```python
from build123d import *

# Parameters (mm, degrees)
SKETCH1_R           = 25.4
BOSS_EXTRUDE1_DEPTH = 10.9
SKETCH4_OUTSIDE_W   = 67.332
SKETCH4_OUTSIDE_H   = 67.332
SKETCH4_OUTSIDE_R   = 23.9
CUT_EXTRUDE3_DEPTH  = 3
SHELL2_T            = -1.5
SKETCH2_R           = 1.7
CUT_EXTRUDE1_DEPTH  = 38.538380359
FILLET1_R           = 3
SKETCH3_R           = 22.5
CUT_EXTRUDE2_DEPTH  = 1.1


with BuildPart() as part:
    # Sketch1 → Boss-Extrude1 (new body)
    with BuildSketch(Plane(origin=(0, 0, 0), x_dir=(1, 0, 0), z_dir=(0, 1, 0))):
        with Locations(Location((0, 0, 0), (0, 0, 270))):
            Circle(SKETCH1_R)
    extrude(amount=BOSS_EXTRUDE1_DEPTH)

    # Sketch4 outside → Cut-Extrude3 (cut)
    with BuildSketch(Plane.XZ):
        Rectangle(SKETCH4_OUTSIDE_W, SKETCH4_OUTSIDE_H)
        with Locations(Location((0, 0, 0), (0, 0, 270))):
            Circle(SKETCH4_OUTSIDE_R, mode=Mode.SUBTRACT)
    extrude(amount=-CUT_EXTRUDE3_DEPTH, mode=Mode.SUBTRACT)

    # Shell2
    shell2_openings = [part.faces().sort_by_distance(p)[0] for p in [
        (0, 0, 0),
    ]]
    offset(amount=SHELL2_T, openings=shell2_openings, kind=Kind.INTERSECTION)

    # Sketch2 → Cut-Extrude1 (cut, through all)
    with BuildSketch(Plane(origin=(0, 10.9, 0), x_dir=(1, 0, 0), z_dir=(0, 1, 0))):
        with Locations(Location((0, 12.375623311, 0), (0, 0, 270))):
            Circle(SKETCH2_R)
        with Locations(Location((8.750887165, 8.750887165, 0), (0, 0, 270))):
            Circle(SKETCH2_R)
        with Locations(Location((12.375623311, 0, 0), (0, 0, 270))):
            Circle(SKETCH2_R)
        with Locations(Location((8.750887165, -8.750887165, 0), (0, 0, 270))):
            Circle(SKETCH2_R)
        with Locations(Location((0, -12.375623311, 0), (0, 0, 270))):
            Circle(SKETCH2_R)
        with Locations(Location((-8.750887165, -8.750887165, 0), (0, 0, 270))):
            Circle(SKETCH2_R)
        with Locations(Location((-12.375623311, 0, 0), (0, 0, 270))):
            Circle(SKETCH2_R)
        with Locations(Location((-8.750887165, 8.750887165, 0), (0, 0, 270))):
            Circle(SKETCH2_R)
    extrude(amount=-CUT_EXTRUDE1_DEPTH, mode=Mode.SUBTRACT)

    # Fillet1
    fillet1_edges = [part.edges().sort_by_distance(p)[0] for p in [
        (0, 10.9, -25.4),
    ]]
    fillet(fillet1_edges, radius=FILLET1_R)

    # Sketch3 → Cut-Extrude2 (cut)
    with BuildSketch(Plane(origin=(0, 10.9, 0), x_dir=(1, 0, 0), z_dir=(0, 1, 0))):
        with Locations(Location((0, 0, 0), (0, 0, 270))):
            Circle(SKETCH3_R)
    extrude(amount=-CUT_EXTRUDE2_DEPTH, mode=Mode.SUBTRACT)


solid = part.part
```
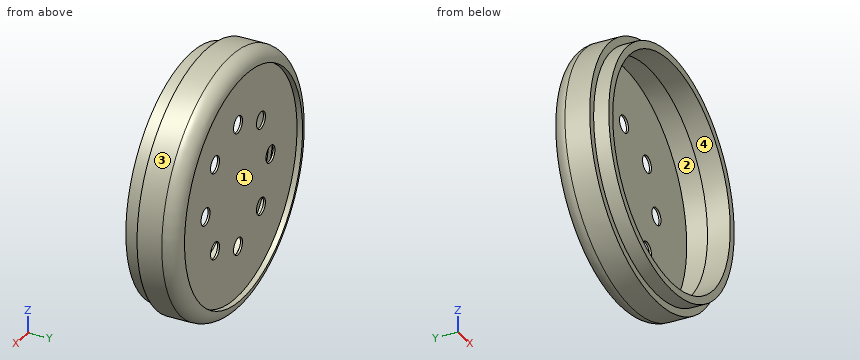
Geometry check sheet. Reference: the model listing, model coordinates, mm. Face numbers are marked on the shaded views. A direction names the side the tool comes from. Coordinates: 2 decimals unless noted, no trailing zeros. Order: outer loops, then holes, each group sorted by start corner. A loop starts at its lowest first (then second) coordinate and runs counter-clockwise, first axis right, second up. Notation, with made-up numbers: (57.5, 69.25) - (109.5, 69.25) arc R12 ccw to (109.5, 77.25) - close; hole circle Ø2 at (-10.5, 73). An arc over 180 degrees is marked (long way). Answer in a Markdown table with one row per item. Add a question column.
1. Draft check along X on the marked faces 3 and 4. Enter one of: +X half, -X half, draft (parallel to the pull), parting line (faces both ways), or undercut.
2. Section check D-D (y = 6.5). Enter the section's corners in (x, z), plus the area to 3 significant figures.
3. Material ranges on L1, parallel to Z at x = 0, y = 7.8; L2, parallel to Y at x = 21.5, z = -6.5; L3, parallel to Y at x = 0.5, z = 8, recorded low to high. Write a range as [from, to].
4. Section check C-C (y = 2.25). Enter the section's corners in (x, z), plus the area to 3 significant figures.
5. Gauge pin test, flat ends, axial feed: pin 1 Ø6 at (x, z) = (-5.5, -6) entering from +Y; pin 2 Ø5.5 at (x, z) = (8.75, 8.75) entering from -Y; pin 3 Ø5 at (x, y) = (13, 5.5) entering from -Z; pin 4 Ø3 at (x, z) = (-8.75, 8.75) entering from -Y. Record the tip position at first contact, or that the pin passes through.
6. Access from +Z, -Z, +X, -X, +Y, -Y to the whole of each face (thin tool, end or side, straight path). Record for the marked faces 1 and 2.
7. Section check A-A (z = 0). Enter the section's corners in (x, y), plus the area to 3 significant figures.
8. Section check B-B (x = 0). Enter the section's corners in (y, z).
Data:
| question | item | result |
|---|---|---|
| 1 | face 3 | parting line |
| 1 | face 4 | undercut |
| 2 | outline | circle Ø50.8 at (0, 0); hole circle Ø47.8 at (0, 0) |
| 2 | area | 232 mm² |
| 3 | L1 | z = [-25.4, -23.9], [23.9, 25.4] |
| 3 | L2 | y = [0, 4.5], [9.4, 9.8] |
| 3 | L3 | y = [9.4, 9.8] |
| 4 | outline | circle Ø47.8 at (0, 0); hole circle Ø44.8 at (0, 0) |
| 4 | area | 218 mm² |
| 5 | pin 1 | stops at y = 9.8 |
| 5 | pin 2 | stops at y = 9.4 |
| 5 | pin 3 | stops at z = -23.13 |
| 5 | pin 4 | passes through |
| 6 | face 1 | +Y |
| 6 | face 2 | none |
| 7 | outline | (-25.4, 3) - (-23.9, 3) - (-23.9, 0) - (-22.4, 0) - (-22.4, 4.5) - (-23.9, 4.5) - (-23.9, 9.4) - (-14.08, 9.4) - (-14.08, 9.8) - (-22.5, 9.8) - (-22.5, 10.9) arc R3 ccw to (-25.4, 7.9) - close; (-10.68, 9.4) - (10.68, 9.4) - (10.68, 9.8) - (-10.68, 9.8) - close; (14.08, 9.4) - (23.9, 9.4) - (23.9, 4.5) - (22.4, 4.5) - (22.4, 0) - (23.9, 0) - (23.9, 3) - (25.4, 3) - (25.4, 7.9) arc R3 ccw to (22.5, 10.9) - (22.5, 9.8) - (14.08, 9.8) - close |
| 7 | area | 52.8 mm² |
| 8 | outline | (0, -23.9) - (3, -23.9) - (3, -25.4) - (7.9, -25.4) arc R3 ccw to (10.9, -22.5) - (9.8, -22.5) - (9.8, -14.08) - (9.4, -14.08) - (9.4, -23.9) - (4.5, -23.9) - (4.5, -22.4) - (0, -22.4) - close; (0, 22.4) - (4.5, 22.4) - (4.5, 23.9) - (9.4, 23.9) - (9.4, 14.08) - (9.8, 14.08) - (9.8, 22.5) - (10.9, 22.5) arc R3 ccw to (7.9, 25.4) - (3, 25.4) - (3, 23.9) - (0, 23.9) - close; (9.4, -10.68) - (9.8, -10.68) - (9.8, 10.68) - (9.4, 10.68) - close |
